```python
from build123d import *

# Parameters (mm, degrees)
SKETCH_R      = 28
SKETCH_R_2    = 15
PAD_DEPTH     = 2
SKETCH003_R   = 22
SKETCH003_R_2 = 16
PAD001_DEPTH  = 0.7
SKETCH002_R   = 2
POCKET_DEPTH  = 2.701


with BuildPart() as part:
    # Sketch → Pad (new body)
    with BuildSketch(Plane.XY):
        Circle(SKETCH_R)
        Circle(SKETCH_R_2, mode=Mode.SUBTRACT)
    extrude(amount=PAD_DEPTH)

    # Sketch003 (on Face4 of Pad) → Pad001 (join)
    with BuildSketch(Plane.XY.offset(2)):
        Circle(SKETCH003_R)
        Circle(SKETCH003_R_2, mode=Mode.SUBTRACT)
    extrude(amount=PAD001_DEPTH)

    # Sketch002 → Pocket (cut, through all)
    with BuildSketch(Plane.XY):
        with Locations((0, 18.5)):
            Circle(SKETCH002_R)
        with Locations((16.02147, -9.25)):
            Circle(SKETCH002_R)
        with Locations((-16.02147, -9.25)):
            Circle(SKETCH002_R)
    extrude(amount=POCKET_DEPTH, mode=Mode.SUBTRACT)


solid = part.part
```
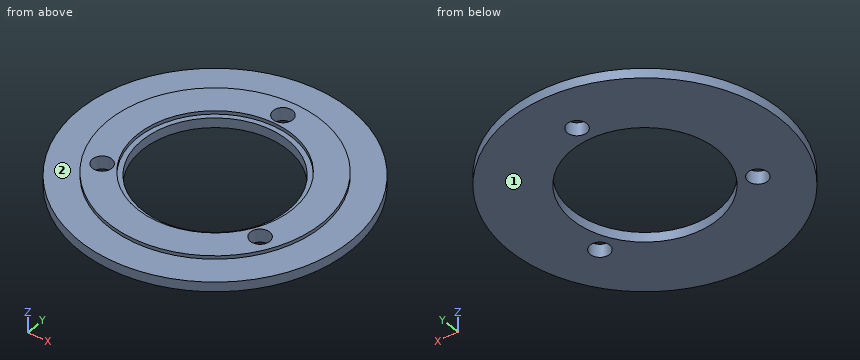
Part model, mm, in its own coordinate system. Face numbers are marked on the shaded views. A direction names the side the tool comes from. Coordinates: 2 decimals unless noted, no trailing zeros. Order: outer loops, then holes, each group sorted by start corner. A loop starts at its lowest first (then second) coordinate and runs counter-clockwise, first axis right, second up. Notation, with made-up numbers: (19, 27.25) - (44, 27.25) arc R20 cw to (44, 57.25) - close; hole circle Ø8 at (24.5, 53.25). An arc over 180 degrees is marked (long way). Return JSON: item names as keys, results as strings. Group by question number.
Item 1: Cut at B-B (y = 0). List the corners of the cut face in (x, z), plus the area to 3 significant figures.
Item 2: Cut at A-A (x = 0). List the corners of the cut face in (y, z), plus the area to 3 significant figures.
Item 3: Drill centre lines: probe 1 along Y at (x, z) = (0, 2.3); probe 2 along Y at (x, z) = (0, 1.2); probe 3 along X at (y, z) = (-9.25, 1.25). Where is each one in solid material? Low to high. Write a range as from..to.
Item 4: Which spindle directions (+Z, -Z, +X, -X, +Y, -Y) get a long thin tool onto all of the face, cutting with end or side? Do the marked faces 1 and 2. Say none if no direction does.
Item 5: Cut at D-D (x = 9.5). List the corners of the cut face in (y, z), plus the area to 3 significant figures.
Item 6: Cut at C-C (z = 0.5). List the corners of the cut face in (x, y).
Item 7: Pin check, flat tips, straight feed: pin 1 (6.5 mm diameter, centred on x = 16.02, y = -9.25, fed in from -Z); pin 2 (1 mm diameter, centred on y = -5.5, z = 1.5, fed in from +X); pin 3 (1 mm diameter, centred on y = 1, z = 0.5, fed in from +X). Stop position of each tip, or through.
Check values:
{
 "1": {"outline": "(-28, 0) - (-15, 0) - (-15, 2) - (-16, 2) - (-16, 2.7) - (-22, 2.7) - (-22, 2) - (-28, 2) - close; (15, 0) - (28, 0) - (28, 2) - (22, 2) - (22, 2.7) - (16, 2.7) - (16, 2) - (15, 2) - close", "area": "60.4 mm2"},
 "2": {"outline": "(-28, 0) - (-15, 0) - (-15, 2) - (-16, 2) - (-16, 2.7) - (-22, 2.7) - (-22, 2) - (-28, 2) - close; (15, 0) - (16.5, 0) - (16.5, 2.7) - (16, 2.7) - (16, 2) - (15, 2) - close; (20.5, 0) - (28, 0) - (28, 2) - (22, 2) - (22, 2.7) - (20.5, 2.7) - close", "area": "49.6 mm2"},
 "3": {"probe 1": "y = -22..-16, 16..16.5, 20.5..22", "probe 2": "y = -28..-15, 15..16.5, 20.5..28", "probe 3": "x = -26.43..-18.02, -14.02..-11.81, 11.81..14.02, 18.02..26.43"},
 "4": {"face 1": "-Z, +X, -X, +Y, -Y", "face 2": "+Z"},
 "5": {"outline": "(-26.34, 0) - (-11.61, 0) - (-11.61, 2) - (-12.87, 2) - (-12.87, 2.7) - (-19.84, 2.7) - (-19.84, 2) - (-26.34, 2) - close; (11.61, 0) - (26.34, 0) - (26.34, 2) - (19.84, 2) - (19.84, 2.7) - (12.87, 2.7) - (12.87, 2) - (11.61, 2) - close", "area": "68.7 mm2"},
 "6": {"outline": "circle Ø56 at (0, 0); hole circle Ø4 at (-16.02, -9.25); hole circle Ø30 at (0, 0); hole circle Ø4 at (0, 18.5); hole circle Ø4 at (16.02, -9.25)"},
 "7": {"pin 1": "stops at z = 0", "pin 2": "stops at x = 27.55", "pin 3": "stops at x = 28"}
}
